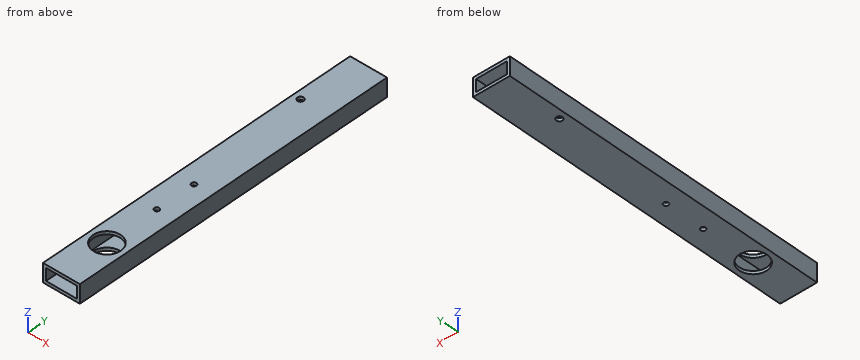
```python
from build123d import *

# Parameters (mm, degrees)
SKETCH1_W           = 38.1
SKETCH1_H           = 19.05
SKETCH1_W_2         = 31.75
SKETCH1_H_2         = 12.7
BOSS_EXTRUDE1_DEPTH = 342.9
SKETCH2_R           = 14.2875
CUT_EXTRUDE1_DEPTH  = 20.05
SKETCH3_R           = 2.54
SKETCH3_R_2         = 3.175
CUT_EXTRUDE2_DEPTH  = 20.05


with BuildPart() as part:
    # Sketch1 → Boss-Extrude1 (new body)
    with BuildSketch(Plane(origin=(0, 0, 0), x_dir=(1, 0, 0), z_dir=(0, 1, 0))):
        with Locations((19.05, 9.525)):
            Rectangle(SKETCH1_W, SKETCH1_H)
        with Locations((19.05, 9.525)):
            Rectangle(SKETCH1_W_2, SKETCH1_H_2, mode=Mode.SUBTRACT)
    extrude(amount=BOSS_EXTRUDE1_DEPTH)

    # Sketch2 → Cut-Extrude1 (cut, through all)
    with BuildSketch(Plane.XY):
        with Locations((19.05, 50.8)):
            Circle(SKETCH2_R)
    extrude(amount=-CUT_EXTRUDE1_DEPTH, mode=Mode.SUBTRACT)

    # Sketch3 → Cut-Extrude2 (cut, through all)
    with BuildSketch(Plane(origin=(0, 0, -19.05), x_dir=(-1, 0, 0), z_dir=(0, 0, -1))):
        with Locations((-19.05, 106.541886393)):
            Circle(SKETCH3_R)
        with Locations((-19.05, 147.996272786)):
            Circle(SKETCH3_R)
        with Locations((-7.946710848, 278.981271676)):
            Circle(SKETCH3_R_2)
    extrude(amount=-CUT_EXTRUDE2_DEPTH, mode=Mode.SUBTRACT)


solid = part.part
```
Work out the finished part from the listing and answer in its coordinate system (mm). Coordinates: 2 decimals unless noted, no trailing zeros. Order: outer loops, then holes, each group sorted by start corner. A loop starts at its lowest first (then second) coordinate and runs counter-clockwise, first axis right, second up. Notation, with made-up numbers: (-0.75, -26.75) - (19.25, -26.75) arc R16 cw to (19.25, -2.75) - close; hole circle Ø3 at (-39.75, -4). An arc over 180 degrees is marked (long way). Answer as a JSON object with one key per item and string values.
1. Consider line 1 (Y direction, x = 19.05, z = -17.75); line 2 (X direction, y = 122, z = -15) (3 decimals); line 3 (Z direction, x = 32, y = 94.5) (3 decimals). Determine where each line is inside the solid, lowest interval first.
Output values:
{"line 1": "y = 0 to 36.51, 65.09 to 104, 109.08 to 145.46, 150.54 to 342.9", "line 2": "x = 0 to 3.175, 34.925 to 38.1", "line 3": "z = -19.05 to -15.875, -3.175 to 0"}
2. This flat-tipped pin is pushed along its axis until it touches: P1, Ø1, axis at x = 10, z = -5.5, coming from the -Y side. Where does it stop, or does it pass through?
Output values:
{"P1": "passes through"}
3. Find section C-C on y = 98. Determine the outline of the cut face in (x, z) (3 decimals).
Output values:
{"outline": "(0, -19.05) - (38.1, -19.05) - (38.1, 0) - (0, 0) - close; hole (3.175, -15.875) - (34.925, -15.875) - (34.925, -3.175) - (3.175, -3.175) - close"}
4. Find section A-A on z = -11.75. Determine the outline of the cut face in (x, y) (3 decimals), plus the area to 3 significant figures.
Output values:
{"outline": "(0, 0) - (3.175, 0) - (3.175, 342.9) - (0, 342.9) - close; (34.925, 0) - (38.1, 0) - (38.1, 342.9) - (34.925, 342.9) - close", "area": "2,180 mm²"}
